Read the model definition and answer for the solid it produces. Units are mm, in the model's axes. A direction names the side the tool comes from. Give positions to 0.01 mm unless a question says otherwise; leave off trailing zeros. Write each loop counter-clockwise with the first axis right and the second up, starting at its lowest first coordinate (ties: lowest second). Pieces come first, ordered by that corner, then holes.
Autodesk Inventor part; units mm, degrees
ref_plane "Start plane" through (0, 0, 0) normal (0, 0, 1) x (1, 0, 0)
ref_plane "End plane" through (0, 0, 651) normal (0, 0, 1) x (1, 0, 0)
ref_plane "YZ Plane" through (0, 0, 0) normal (1, 0, 0) x (0, 1, 0)
ref_plane "Start plane" through (0, 0, 0) normal (0, 0, 1) x (1, 0, 0)
ref_plane "End plane" through (0, 0, 651) normal (0, 0, 1) x (1, 0, 0)
sketch "Sketch" plane through (0, 0, 0) normal (0, 0, 1) x (1, 0, 0)
  line L0 (-9.2, 25) -> (9.2, 25)
  line L1 (15, 19.2) -> (15, -19.2)
  line L2 (9.2, -25) -> (-9.2, -25)
  line L3 (-15, -19.2) -> (-15, 19.2)
  arc A0 (-9.2, 25) -> (-15, 19.2) centre (-9.2, 19.2) ccw
  arc A1 (15, 19.2) -> (9.2, 25) centre (9.2, 19.2) ccw
  arc A2 (9.2, -25) -> (15, -19.2) centre (9.2, -19.2) ccw
  arc A3 (-15, -19.2) -> (-9.2, -25) centre (-9.2, -19.2) ccw
  line L4 (-22.6817, 0) -> (22.6817, 0) construction
  line L5 (0, -36.6817) -> (0, 36.6817) construction
  arc A4 (-9.2, 22.1) -> (-12.1, 19.2) centre (-9.2, 19.2) ccw
  line L6 (-9.2, 22.1) -> (9.2, 22.1)
  arc A5 (12.1, 19.2) -> (9.2, 22.1) centre (9.2, 19.2) ccw
  line L7 (12.1, 19.2) -> (12.1, -19.2)
  arc A6 (9.2, -22.1) -> (12.1, -19.2) centre (9.2, -19.2) ccw
  line L8 (9.2, -22.1) -> (-9.2, -22.1)
  arc A7 (-12.1, -19.2) -> (-9.2, -22.1) centre (-9.2, -19.2) ccw
  line L9 (-12.1, -19.2) -> (-12.1, 19.2)
  point P0 (-15, 25)
  point P1 (15, -25)
  point P2 (15, 25)
  dimension "b" = 30
  dimension "ParH" = 50
  dimension "msp_r" = 5.8
  dimension "d8" = 15
  dimension "d9" = 25
  dimension "d10" = 2.9
extrude "Body" add sketch "Sketch" along normal up to surface (651 mm away) from surface at 0
sketch "Sketch2" plane through (0, 0, 0) normal (0, 0, 1) x (1, 0, 0)
  line L0 (0, 0) -> (10, 0)
ref_plane "Work Plane3" through (0, 0, 0) normal (0, -1, 0) x (1, 0, 0)
sketch "Sketch3" plane through (0, 0, 0) normal (0, -1, 0) x (1, 0, 0)
  line L0 (-2, 0) -> (12, 0)
  line L1 (-2, 651) -> (12, 651)
  dimension "d14" = 651
equation "\"msp_r\" = 2 * ParT"
equation "\"d8\" = 0.5 * b"
equation "\"d9\" = 0.5 * ParH"
equation "\"d10\" = ParT"
equation "\"G_OFFSET_START\" = 0"
equation "\"G_OFFSET_END\" = 0"
equation "\"d12\" = G_OFFSET_END + B_L"
equation "\"G_L\" = d14"
equation "\"B_L\" = 651"
properties part number "DIN 59 410 - 50x30x2.9-651" material "Steel, Mild"
Item 1: Find the intervals of material crossed by line 1 along X through (y, z) = (10.5, 30); line 2 along Y through (x, z) = (6.25, 381); line 3 along Y through (x, z) = (11, 576), in increasing order.
Result set:
line 1: x = -15 to -12.1, 12.1 to 15
line 2: y = -25 to -22.1, 22.1 to 25
line 3: y = -24.71 to -21.47, 21.47 to 24.71
Item 2: Section B-B (y = 11) is taken. Write down the section's boundary in (x, z), and give its area (3 significant figures).
Result set:
outline: (-15, 0) - (-12.1, 0) - (-12.1, 651) - (-15, 651) - close; (12.1, 0) - (15, 0) - (15, 651) - (12.1, 651) - close
area: 3,780 mm2
Item 3: Section C-C (z = 583.5) is taken. Write down the section's boundary in (x, y).
Result set:
outline: (-15, -19.2) arc R5.8 ccw to (-9.2, -25) - (9.2, -25) arc R5.8 ccw to (15, -19.2) - (15, 19.2) arc R5.8 ccw to (9.2, 25) - (-9.2, 25) arc R5.8 ccw to (-15, 19.2) - close; hole (-12.1, -19.2) arc R2.9 ccw to (-9.2, -22.1) - (9.2, -22.1) arc R2.9 ccw to (12.1, -19.2) - (12.1, 19.2) arc R2.9 ccw to (9.2, 22.1) - (-9.2, 22.1) arc R2.9 ccw to (-12.1, 19.2) - close
Item 4: Which of the six approach directions +Z, -Z, +X, -X, +Y, -Y give full straight-line access (tool end or side, diameter ignored) to faces 4 (the flat face through (12.1, 0, 321)), 5 (the flat face through (15, 0, 321))?
Result set:
face 4: +Z, -Z
face 5: +Z, -Z, +X, +Y, -Y
Item 5: Determine the mould class of faces 1 (the flat face through (-15, 0, 321)), 2 (the flat face through (0, 22.1, 321)), 3 (the flat face through (-12.3, 2, 0)) for opening direction X: pulls with the +X half, pulls with the -X half, needs draft (parallel to the pull), parting line crosses it, or undercut.
Result set:
face 1: pulls with the -X half
face 2: undercut
face 3: needs draft
Item 6: Section A-A (x = -0.5) is taken. Write down the section's boundary in (y, z), and give its area (3 significant figures).
Result set:
outline: (-25, 0) - (-22.1, 0) - (-22.1, 651) - (-25, 651) - close; (22.1, 0) - (25, 0) - (25, 651) - (22.1, 651) - close
area: 3,780 mm2
